Job drawing, mm, ordinate dimensions from the low corner. One solid piece. A direction names the side the tool comes from. Give positions to 0.01 mm unless a question says otherwise; leave off trailing zeros. Write each loop counter-clockwise with the first axis right and the second up, starting at its lowest first coordinate (ties: lowest second). Pieces come first, ordered by that corner, then holes. Notation, with made-up numbers: M 82.5,78.25 L 130.5,78.25 A20 ccw 130.5,89.25 Z; hole C -10.75,78.5 d8. An arc over 180 degrees is marked long. Use a Markdown table: item, result.
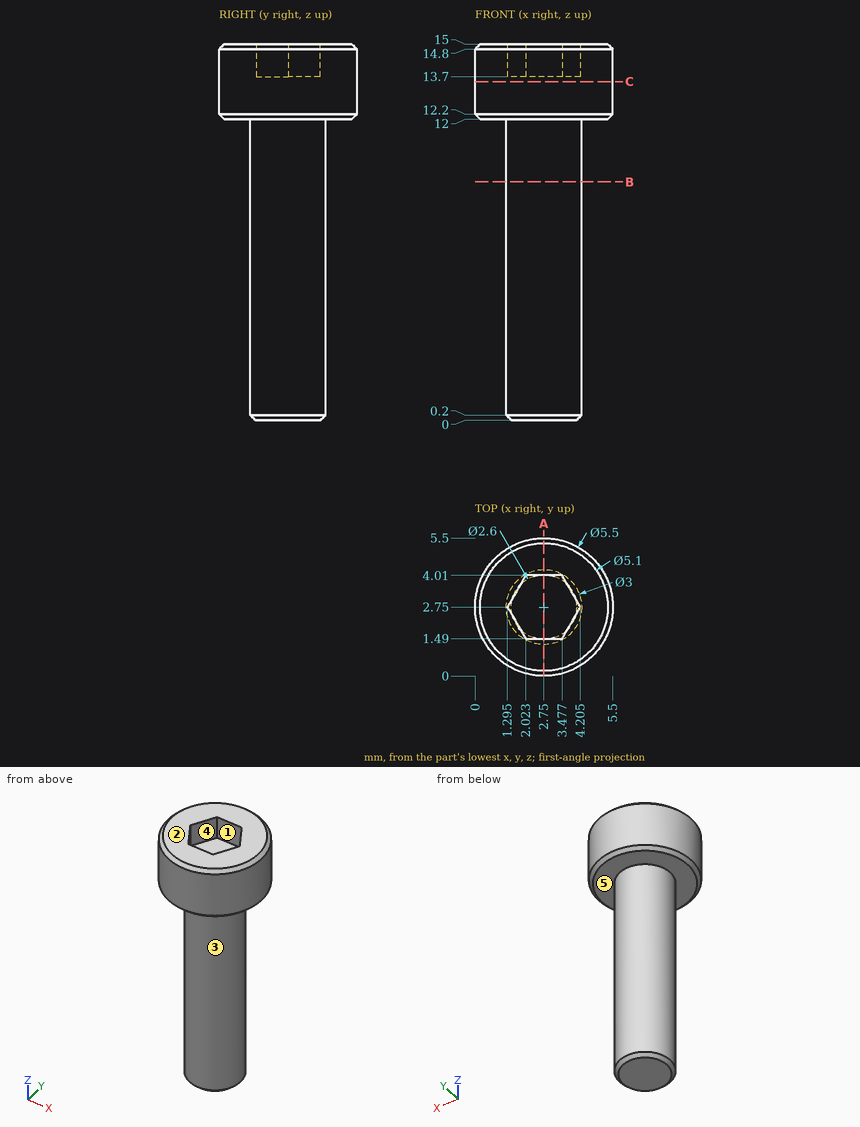
1. Two-plate mould, pull along Y, no slides. Class the marked faces 3, 4 and 5: released by +Y, released by -Y, zero draft, split by the parting line, or undercut.
Findings below:
| item | result |
|---|---|
| face 3 | split by the parting line |
| face 4 | undercut |
| face 5 | zero draft |
2. Cut at A-A, the plane x = 2.75. Give the cut face in (y, z), then the cut area to 3 significant figures.
Findings below:
| item | result |
|---|---|
| outline | M 0,12.2 L 0.2,12 L 1.25,12 L 1.25,0.2 L 1.45,0 L 4.05,0 L 4.25,0.2 L 4.25,12 L 5.3,12 L 5.5,12.2 L 5.5,14.8 L 5.3,15 L 4.01,15 L 4.01,13.7 L 1.49,13.7 L 1.49,15 L 0.2,15 L 0,14.8 Z |
| area | 49.1 mm2 |
3. Drop flat-ended pins along their axis: P1, Ø3, axis at x = 1, z = 12, coming from the -Y side; P2, Ø1, axis at x = 2, z = 12.5, coming from the +Y side; P3, Ø2, axis at y = 3, z = 2, coming from the +X side. Give the stop position or say it passes through.
Findings below:
| item | result |
|---|---|
| P1 | y = 0.01 |
| P2 | y = 5.49 |
| P3 | x = 4.25 |
4. Tool access for the marked faces 1 and 2: list every direction of +Z, -Z, +X, -X, +Y, -Y with a clear straight run to the whole face (end or side of a thin tool).
Findings below:
| item | result |
|---|---|
| face 1 | +Z |
| face 2 | +Z, +X, -X, +Y, -Y |
5. Cut at C-C, the plane z = 13.5. Give the cut face in (x, y).
Findings below:
| item | result |
|---|---|
| outline | C 2.75,2.75 d5.5 |
6. Cut at B-B, the plane z = 9.5. Give the cut face in (x, y).
Findings below:
| item | result |
|---|---|
| outline | C 2.75,2.75 d3 |
7. Drill centre lines: L1, parallel to Z at x = 2.45, y = 1.9; L2, parallel to Y at x = 2, z = 4.5; L3, parallel to Z at x = 1.8, y = 0.75. Where is each one in solid material? Low to high.
Findings below:
| item | result |
|---|---|
| L1 | 0 to 13.7 |
| L2 | 1.45 to 4.05 |
| L3 | 12 to 15 |
